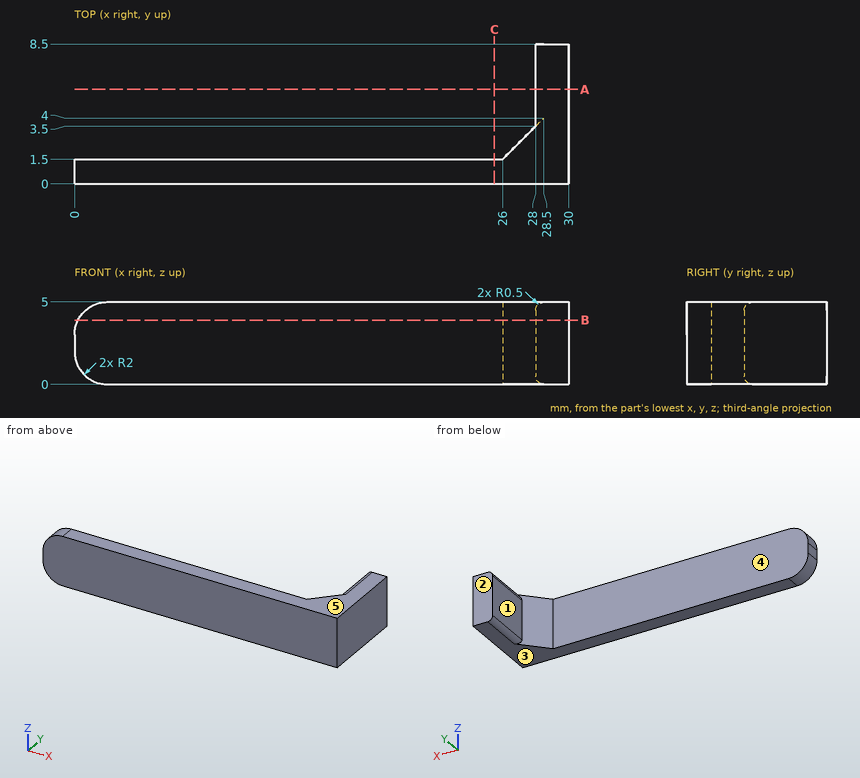
Design review of the part shown in the three views and the two pictorial views. Dimensions are in mm from the part's minimum x, y and z. A direction names the side the tool comes from. Coordinates: 2 decimals unless noted, no trailing zeros. Loops run counter-clockwise (first coordinate to the right, second up) from the corner with the lowest first, then second, coordinate; pieces in that order, holes last. Notation, with made-up numbers: M 57,6 L 104,6 A18 ccw 104,16 Z; hole C -25.5,32 d5. An arc over 180 degrees is marked long. One line per question, with ' | ' between items.
(1) We need section A-A (y = 5.75). Give the boundary of the cut face in (x, z).
Filled in:
outline: M 28,0.5 A0.5 ccw 28.5,0 L 30,0 L 30,5 L 28.5,5 A0.5 ccw 28,4.5 Z
(2) For pin 1 Ø2 at (y, z) = (4, 1) entering from -X; pin 2 Ø1.5 at (y, z) = (5.5, 2.5) entering from -X, all flat-tipped, find the tip position at first contact; note any pin that passes through.
Filled in:
pin 1: stops at x = 27.5 | pin 2: stops at x = 28
(3) Machinability: for the marked faces 1 and 2, which of the approach directions +Z, -Z, +X, -X, +Y, -Y give a long, thin tool a straight path to every point of the face, cutting with its end or side? Answer none if there is none.
Filled in:
face 1: +Z, -Z, -X, +Y | face 2: +Z, -Z, +X, -X, +Y
(4) We need section B-B (z = 3.9). Give the boundary of the cut face in (x, y).
Filled in:
outline: M 0.21,0 L 30,0 L 30,8.5 L 28,8.5 L 28,3.5 L 26,1.5 L 0.21,1.5 Z
(5) Wall thickness on probe 1 along X at (y, z) = (5, 4.45); probe 2 along Y at (x, z) = (10.25, 3.5); probe 3 along X at (y, z) = (2.25, 3.7): over which ranges is each line inside the solid? List them lowest first.
Filled in:
probe 1: x = 28 to 30 | probe 2: y = 0 to 1.5 | probe 3: x = 26.75 to 30
(6) We need section C-C (x = 25.5). Give the boundary of the cut face in (y, z), and give its area (3 significant figures).
Filled in:
outline: M 0,0 L 1.5,0 L 1.5,5 L 0,5 Z | area: 7.50 mm^2
(7) Draft analysis for pull direction Z (two halves, no side actions). For the marked faces 3, 4 and 5, state which applies: released by +Z, released by -Z, zero draft, split by the parting line, or undercut.
Filled in:
face 3: released by -Z | face 4: zero draft | face 5: released by +Z
